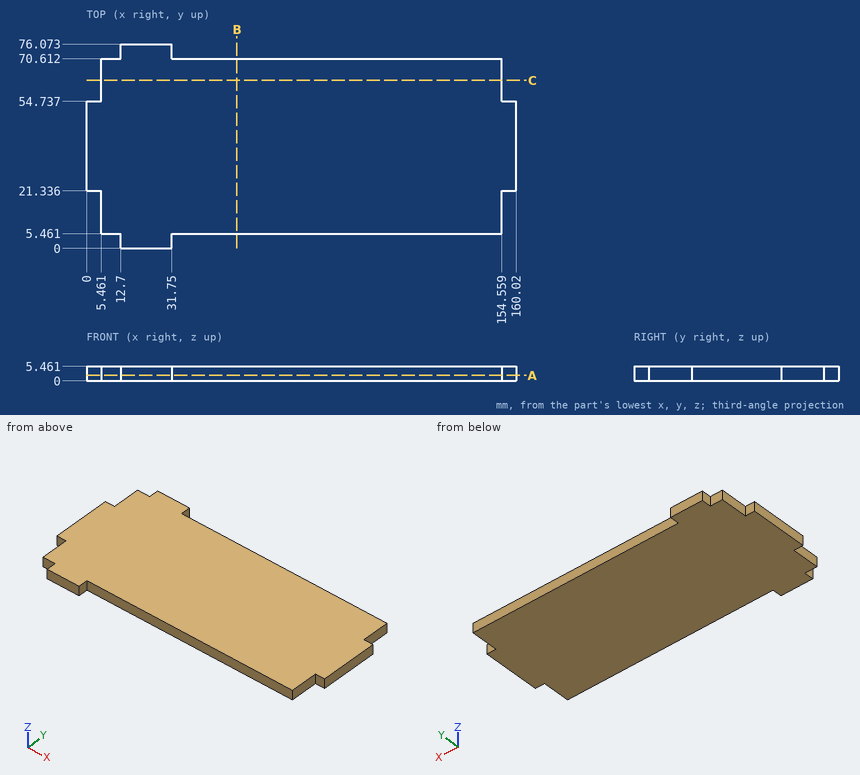
Job drawing, mm, ordinate dimensions from the low corner. One solid piece. Coordinates: 2 decimals unless noted, no trailing zeros. Write each loop counter-clockwise with the first axis right and the second up, starting at its lowest first coordinate (ties: lowest second). Pieces come first, ordered by that corner, then holes.
Item 1: Pin check, flat tips, straight feed: pin 1 (1.6 mm diameter, centred on x = 2, z = 1.5, fed in from +Y); pin 2 (2.5 mm diameter, centred on x = 10.5, z = 2, fed in from +Y); pin 3 (3 mm diameter, centred on x = 107.5, z = 3, fed in from -Y). Stop position of each tip, or through.
Item 2: Slice it at A-A (z = 2.05). Write the cut outline in (x, y), and give its area (3 significant figures).
Item 3: Slice it at B-B (x = 56). Write the cut outline in (y, z).
Item 4: Probe line 1 (X direction, y = 14, z = 3.2); line 2 (Y direction, x = 88.5, z = 1.25); line 3 (X direction, y = 71.5, z = 1.6). List the from-to ranges inside material, lowest first.
Item 5: Slice it at C-C (y = 62.5). Write the cut outline in (x, z).
Results found:
1. pin 1: stops at y = 54.74
1. pin 2: stops at y = 70.61
1. pin 3: stops at y = 5.46
2. outline: (0, 21.34) - (5.46, 21.34) - (5.46, 5.46) - (12.7, 5.46) - (12.7, 0) - (31.75, 0) - (31.75, 5.46) - (154.56, 5.46) - (154.56, 21.34) - (160.02, 21.34) - (160.02, 54.74) - (154.56, 54.74) - (154.56, 70.61) - (31.75, 70.61) - (31.75, 76.07) - (12.7, 76.07) - (12.7, 70.61) - (5.46, 70.61) - (5.46, 54.74) - (0, 54.74) - close
2. area: 10,300 mm2
3. outline: (5.46, 0) - (70.61, 0) - (70.61, 5.46) - (5.46, 5.46) - close
4. line 1: x = 5.46 to 154.56
4. line 2: y = 5.46 to 70.61
4. line 3: x = 12.7 to 31.75
5. outline: (5.46, 0) - (154.56, 0) - (154.56, 5.46) - (5.46, 5.46) - close
